Work out the finished part from the listing and answer in its coordinate system (mm). Coordinates: 2 decimals unless noted, no trailing zeros. Order: outer loops, then holes, each group sorted by start corner. A loop starts at its lowest first (then second) coordinate and runs counter-clockwise, first axis right, second up.
1. The part is cut by section B-B, the plane x = 0. Give the vertices of the cut face in (y, z).
2. Find the intervals of material crossed by probe 1 along X at (y, z) = (0, 5); probe 2 along X at (y, z) = (3.75, 4.25), in increasing order.
3. The part is cut by section C-C, the plane z = 7.5. Give the vertices of the cut face in (x, y).
4. The part is cut by section A-A, the plane y = -9.75. Give the vertices of the cut face in (x, z).
5. The part is cut by section D-D, the plane z = 4.75. Give the vertices of the cut face in (x, y).
6. Flat-ended cylindrical pins translate along their axes: pin 1 Ø1.5 at (y, z) = (-7.5, 6.5) entering from +X; pin 2 Ø3 at (y, z) = (11, 4.5) entering from -X; pin 3 Ø1 at (x, z) = (6, 8.5) entering from +Y. Find the tip coordinate at first contact, or state that the pin passes through.
```python
from build123d import *

# Parameters (mm, degrees)
SKETCH1_R           = 15
SKETCH1_R_2         = 12.5
BOSS_EXTRUDE1_DEPTH = 10
CUT_EXTRUDE1_DEPTH  = 10


with BuildPart() as part:
    # Sketch1 → Boss-Extrude1 (new body)
    with BuildSketch(Plane.XY):
        Circle(SKETCH1_R)
        Circle(SKETCH1_R_2, mode=Mode.SUBTRACT)
    extrude(amount=BOSS_EXTRUDE1_DEPTH)

    # Sketch2 → Cut-Extrude1 (cut)
    with BuildSketch(Plane(origin=(0, 15, 0), x_dir=(1, 0, 0), z_dir=(0, 1, 0))):
        Polygon((0.693116527, 3.154438347), (-4.706995906, -12.228203461), (-3.793236096, -12.355616729), (1.606876337, 3.02702508), align=None)
    extrude(amount=-CUT_EXTRUDE1_DEPTH, mode=Mode.SUBTRACT)


solid = part.part
```
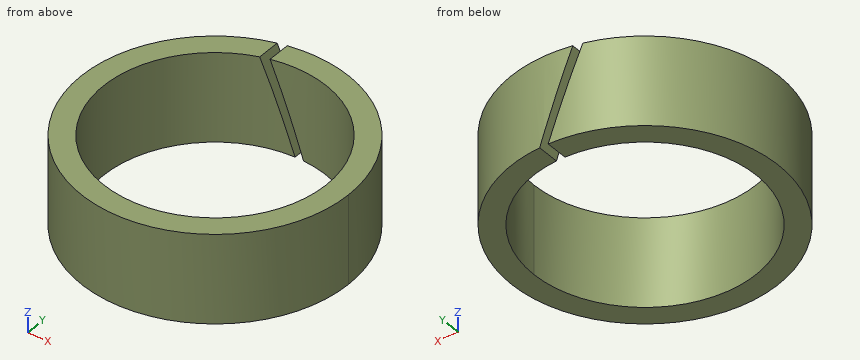
Geometry says:
1. outline: (-15, 0) - (-12.5, 0) - (-12.5, 10) - (-15, 10) - close; (12.5, 1.55) - (15, 1.55) - (15, 10) - (12.5, 10) - close
2. probe 1: x = -15 to -12.5, 12.5 to 15
2. probe 2: x = -14.52 to -11.92, 11.92 to 14.52
3. outline: (-3.05, 12.12) - (-3.05, 14.69) arc R15 ccw (long way) to (-2.09, 14.85) - (-2.09, 12.32) arc R12.5 cw (long way) to start
4. outline: (-11.4, 0) - (-7.82, 0) - (-7.82, 10) - (-11.4, 10) - close; (7.82, 0) - (11.4, 0) - (11.4, 10) - (7.82, 10) - close
5. outline: (-2.08, 12.33) - (-2.08, 14.85) arc R15 ccw (long way) to (-1.12, 14.96) - (-1.12, 12.45) arc R12.5 cw (long way) to start
6. pin 1: stops at x = 13.4
6. pin 2: stops at x = -11.61
6. pin 3: stops at y = 13.96
